```python
from build123d import *

# Parameters (mm, degrees)
SKETCH1_R           = 2.5
BOSS_EXTRUDE1_DEPTH = 20
SKETCH2_W           = 30.1
SKETCH2_H           = 82.1
CUT_EXTRUDE1_DEPTH  = 8.5
SKETCH3_W           = 30.1
SKETCH3_H           = 82.1
CUT_EXTRUDE2_DEPTH  = 6.5
CUT_EXTRUDE3_REACH  = 200.842
SKETCH5_R           = 2.1


with BuildPart() as part:
    # Sketch1 → Boss-Extrude1 (new body)
    with BuildSketch(Plane(origin=(0, 0, 0), x_dir=(1, 0, 0), z_dir=(0, 1, 0))):
        with BuildLine():
            Line((60.104076401, -60.104076401), (46.450402953, -82.609312867))
            ThreePointArc((46.450402953, -82.609312867), (45.36942446, -85.103300576), (45, -87.796257086))
            Line((45, -87.796257086), (45, -118.89))
            Line((45, -118.89), (45, -169.39))
            ThreePointArc((45, -169.39), (42.071067812, -176.461067812), (35, -179.39))
            Line((35, -179.39), (-35, -179.39))
            ThreePointArc((-35, -179.39), (-42.071067812, -176.461067812), (-45, -169.39))
            Line((-45, -169.39), (-45, -118.89))
            Line((-45, -118.89), (-45, -87.796257086))
            ThreePointArc((-45, -87.796257086), (-45.36942446, -85.103300576), (-46.450402953, -82.609312867))
            Line((-46.450402953, -82.609312867), (-60.104076401, -60.104076401))
            ThreePointArc((-60.104076401, -60.104076401), (0, 85), (60.104076401, -60.104076401))
        make_face()
        with Locations(Location((0, 41.5, 0), (0, 0, 270))):
            Circle(SKETCH1_R, mode=Mode.SUBTRACT)
        with Locations(Location((41.5, 0, 0), (0, 0, 270))):
            Circle(SKETCH1_R, mode=Mode.SUBTRACT)
        with Locations(Location((0, -41.5, 0), (0, 0, 270))):
            Circle(SKETCH1_R, mode=Mode.SUBTRACT)
        with Locations(Location((-41.5, 0, 0), (0, 0, 270))):
            Circle(SKETCH1_R, mode=Mode.SUBTRACT)
    extrude(amount=BOSS_EXTRUDE1_DEPTH)

    # Sketch2 → Cut-Extrude1 (cut)
    with BuildSketch(Plane(origin=(0, 20, 0), x_dir=(1, 0, 0), z_dir=(0, 1, 0))):
        with Locations((0, -138.34)):
            Rectangle(SKETCH2_W, SKETCH2_H)
    extrude(amount=-CUT_EXTRUDE1_DEPTH, mode=Mode.SUBTRACT)

    # Sketch3 → Cut-Extrude2 (cut)
    with BuildSketch(Plane.XZ):
        with Locations((0, 138.34)):
            Rectangle(SKETCH3_W, SKETCH3_H)
    extrude(amount=-CUT_EXTRUDE2_DEPTH, mode=Mode.SUBTRACT)

    # Sketch5 → Cut-Extrude3 (cut, up to next)
    with BuildSketch(Plane(origin=(0, 11.5, 0), x_dir=(1, 0, 0), z_dir=(0, 1, 0)), mode=Mode.PRIVATE) as cut_extrude3_sk1:
        with Locations(Location((-8.5, -100.8, 0), (0, 0, 270))):
            Circle(SKETCH5_R)
    cut_extrude3_tool1 = extrude(cut_extrude3_sk1.sketch, amount=-CUT_EXTRUDE3_REACH, mode=Mode.PRIVATE) & part.part
    # Sketch5 → Cut-Extrude3 (cut, up to next)
    with BuildSketch(Plane(origin=(0, 11.5, 0), x_dir=(1, 0, 0), z_dir=(0, 1, 0)), mode=Mode.PRIVATE) as cut_extrude3_sk2:
        with Locations(Location((8.5, -100.8, 0), (0, 0, 270))):
            Circle(SKETCH5_R)
    cut_extrude3_tool2 = extrude(cut_extrude3_sk2.sketch, amount=-CUT_EXTRUDE3_REACH, mode=Mode.PRIVATE) & part.part
    # Sketch5 → Cut-Extrude3 (cut, up to next)
    with BuildSketch(Plane(origin=(0, 11.5, 0), x_dir=(1, 0, 0), z_dir=(0, 1, 0)), mode=Mode.PRIVATE) as cut_extrude3_sk3:
        with Locations(Location((8.5, -175.88, 0), (0, 0, 90))):
            Circle(SKETCH5_R)
    cut_extrude3_tool3 = extrude(cut_extrude3_sk3.sketch, amount=-CUT_EXTRUDE3_REACH, mode=Mode.PRIVATE) & part.part
    # Sketch5 → Cut-Extrude3 (cut, up to next)
    with BuildSketch(Plane(origin=(0, 11.5, 0), x_dir=(1, 0, 0), z_dir=(0, 1, 0)), mode=Mode.PRIVATE) as cut_extrude3_sk4:
        with Locations(Location((-8.5, -175.88, 0), (0, 0, 90))):
            Circle(SKETCH5_R)
    cut_extrude3_tool4 = extrude(cut_extrude3_sk4.sketch, amount=-CUT_EXTRUDE3_REACH, mode=Mode.PRIVATE) & part.part
    add(cut_extrude3_tool1.solids().sort_by_distance((-8.5, 11.5, 100.8))[0], mode=Mode.SUBTRACT)
    add(cut_extrude3_tool2.solids().sort_by_distance((8.5, 11.5, 100.8))[0], mode=Mode.SUBTRACT)
    add(cut_extrude3_tool3.solids().sort_by_distance((8.5, 11.5, 175.88))[0], mode=Mode.SUBTRACT)
    add(cut_extrude3_tool4.solids().sort_by_distance((-8.5, 11.5, 175.88))[0], mode=Mode.SUBTRACT)


solid = part.part
```
Model file for the job. Use its own axes, mm. A direction names the side the tool comes from. Give positions to 0.01 mm unless a question says otherwise; leave off trailing zeros. Order: outer loops, then holes, each group sorted by start corner. A loop starts at its lowest first (then second) coordinate and runs counter-clockwise, first axis right, second up.
1) Saw through at B-B, the plane z = 50. Write the cut outline in (x, y).
2) Saw through at A-A, the plane y = 16.5. Write the cut outline in (x, z).
3) 3-axis set-ups, long thin cutter, end or side, ignore diameter. For faces 4 (the flat face through (0, 6.5, 139)), 5 (the flat face through (45, 10, 128)), 6 (the flat face through (-45, 10, 129)), 7 (the flat face through (-15.05, 16, 139)): which of +Z, -Z, +X, -X, +Y, -Y reach the whole face in a straight line?
4) Mould opens along Z. For faces 1 (the flat face through (0, 3, 97.29)), 2 (the flat face through (15.05, 3, 138)), 3 (the cylindrical face through (-0.96, 9.86, 43.81)) say: +Z half, -Z half, draft (parallel to the pull), parting line (faces both ways), or undercut.
5) Wall check: probe 1 along X at (y, z) = (8, 100.8); probe 2 along X at (y, z) = (7.9, 175.88); probe 3 along X at (y, z) = (4.5, 119). Give the ranges that are in metal, low to high.
6) Pin check, flat tips, straight feed: pin 1 (5 mm diameter, centred on x = 8.5, z = 100.8, fed in from -Y); pin 2 (10 mm diameter, centred on y = 13, z = 145.5, fed in from +X); pin 3 (4 mm diameter, centred on x = 0, z = 41.5, fed in from -Y); pin 4 (12 mm diameter, centred on x = -26.5, y = 16, fed in from -Z). Stop position of each tip, or through.
Computed:
1. outline: (-68.74, 0) - (68.74, 0) - (68.74, 20) - (-68.74, 20) - close
2. outline: (-60.1, 60.1) arc R85 ccw (long way) to (60.1, 60.1) - (46.45, 82.61) arc R10 cw to (45, 87.8) - (45, 169.39) arc R10 ccw to (35, 179.39) - (15.05, 179.39) - (15.05, 97.29) - (-15.05, 97.29) - (-15.05, 179.39) - (-35, 179.39) arc R10 ccw to (-45, 169.39) - (-45, 87.8) arc R10 cw to (-46.45, 82.61) - close; hole circle Ø5 at (-41.5, 0); hole circle Ø5 at (0, -41.5); hole circle Ø5 at (0, 41.5); hole circle Ø5 at (41.5, 0)
3. face 4: +Z, -Y
3. face 5: +Z, +X, +Y, -Y
3. face 6: +Z, -X, +Y, -Y
3. face 7: +Z, +Y
4. face 1: +Z half
4. face 2: draft
4. face 3: undercut
5. probe 1: x = -45 to -10.6, -6.4 to 6.4, 10.6 to 45
5. probe 2: x = -42.61 to -10.6, -6.4 to 6.4, 10.6 to 42.61
5. probe 3: x = -45 to -15.05, 15.05 to 45
6. pin 1: stops at y = 6.5
6. pin 2: stops at x = 45
6. pin 3: passes through
6. pin 4: stops at z = -82.49
